Part model, mm, in its own coordinate system. A direction names the side the tool comes from. Give positions to 0.01 mm unless a question says otherwise; leave off trailing zeros. Write each loop counter-clockwise with the first axis right and the second up, starting at its lowest first coordinate (ties: lowest second). Pieces come first, ordered by that corner, then holes.
from build123d import *

# Parameters (mm, degrees)
SKETCH_1_R                              = 19
HOUSING_OD38_L34_FROM_DRAWING_DEPTH     = 34
SKETCH_2_R                              = 10
PILOT_OD20_L5_DEPTH                     = 5
SKETCH_3_R                              = 5
SIDE_CABLE_GLAND_ENVELOPE_EST_DEPTH     = 5
SKETCH_4_R                              = 1.25
FRONT_3XM3_PCD30_DEPTH6_REFERENCE_DEPTH = 6


with BuildPart() as part:
    # 草图1 → Housing_OD38_L34_from_drawing (new body)
    with BuildSketch(Plane.XY.offset(-34)):
        Circle(SKETCH_1_R)
    extrude(amount=HOUSING_OD38_L34_FROM_DRAWING_DEPTH)

    # 草图2 → Pilot_OD20_L5 (add)
    with BuildSketch(Plane.XY):
        Circle(SKETCH_2_R)
    extrude(amount=PILOT_OD20_L5_DEPTH)

    # 草图3 → Side_cable_gland_ENVELOPE_EST (add)
    with BuildSketch(Plane(origin=(-22, 0, 0), x_dir=(0, 0, -1), z_dir=(1, 0, 0))):
        with Locations(Location((26.5, 0, 0), (0, 0, 180))):
            Circle(SKETCH_3_R)
    extrude(amount=SIDE_CABLE_GLAND_ENVELOPE_EST_DEPTH)

    # 草图4 → Front_3xM3_PCD30_depth6_reference (cut)
    with BuildSketch(Plane.XY):
        with Locations((15, 0)):
            Circle(SKETCH_4_R)
        with Locations((-7.5, 12.990381057)):
            Circle(SKETCH_4_R)
        with Locations((-7.5, -12.990381057)):
            Circle(SKETCH_4_R)
    extrude(amount=-FRONT_3XM3_PCD30_DEPTH6_REFERENCE_DEPTH, mode=Mode.SUBTRACT)


solid = part.part
1) 3-axis set-ups, long thin cutter, end or side, ignore diameter. For faces 1 (the flat face through (0, 0, 5)), 2 (the cylindrical face through (-20.19, -1.5, -21.73)), 3 (the cylindrical face through (-8.75, -12.94, -2.96)): which of +Z, -Z, +X, -X, +Y, -Y reach the whole face in a straight line?
Check result:
face 1: +Z, +X, -X, +Y, -Y
face 2: -X
face 3: +Z
2) Saw through at D-D (x = 15). Write the cut outline in (y, z).
Check result:
outline: (-11.66, -34) - (11.66, -34) - (11.66, 0) - (1.25, 0) - (1.25, -6) - (-1.25, -6) - (-1.25, 0) - (-11.66, 0) - close
3) Saw through at C-C (z = -8). Write the cut outline in (x, y).
Check result:
outline: circle Ø38 at (0, 0)
4) Saw through at A-A (x = 0). Write the cut outline in (y, z).
Check result:
outline: (-19, -34) - (19, -34) - (19, 0) - (10, 0) - (10, 5) - (-10, 5) - (-10, 0) - (-19, 0) - close
5) Saw through at B-B (y = 0). Write the cut outline in (x, z).
Check result:
outline: (-22, -31.5) - (-19, -31.5) - (-19, -34) - (19, -34) - (19, 0) - (16.25, 0) - (16.25, -6) - (13.75, -6) - (13.75, 0) - (10, 0) - (10, 5) - (-10, 5) - (-10, 0) - (-19, 0) - (-19, -21.5) - (-22, -21.5) - close
6) Drill centre lines: L1, parallel to Y at x = -7.5, z = -1.75; L2, parallel to Z at x = -12.5, y = 9; L3, parallel to X at y = -12.5, z = -1.5. Where is each one in solid material? Low to high.
Check result:
L1: y = -17.46 to -14.24, -11.74 to 11.74, 14.24 to 17.46
L2: z = -34 to 0
L3: x = -14.31 to -8.65, -6.35 to 14.31
7) Mould opens along X. For faces 4 (the flat face through (0, 0, -34)), 5 (the cylindrical face through (-8.75, 13.05, -2.96)), 6 (the cylindrical face through (-2.17, -9.76, 2.46)), 7 (the cylindrical face through (13.75, 0.05, -2.96)) say: +X half, -X half, draft (parallel to the pull), parting line (faces both ways), or undercut.
Check result:
face 4: draft
face 5: undercut
face 6: parting line
face 7: undercut
8) Flat gauge pins, fed straight in: P1, Ø12, axis at x = -2.5, z = -21.5, coming from the +Y side; P2, Ø8, axis at y = 10, z = -16.5, coming from the +X side; P3, Ø10, axis at x = -8, z = -2.5, coming from the +Y side. Where does each tip first touch, or does it go through?
Check result:
P1: stops at y = 19
P2: stops at x = 18.03
P3: stops at y = 18.76
